```python
from build123d import *

# Parameters (mm, degrees)
F0_W     = 5.5
F0_H     = 3.5
F1_DEPTH = 4
F2_DEPTH = 8.5
F3_DEPTH = 1


with BuildPart() as f1:
    # F0 (on Front) → F1 (new body)
    with BuildSketch(Plane.XZ):
        Polygon((-5.5, 14.5), (-26.5, 14.5), (-26.5, -14.5), (26.5, -14.5), (26.5, 14.5), (5.5, 14.5), (5.5, 11), (23, 11), (23, -11), (-23, -11), (-23, 11), (-5.5, 11), align=None)
        with Locations((-2.75, 12.75)):
            Rectangle(F0_W, F0_H)
        with Locations((2.75, 12.75)):
            Rectangle(F0_W, F0_H)
        Polygon((0, 11), (-5.5, 11), (-5.5, 6), (5.5, 6), (5.5, 11), align=None)
    extrude(amount=F1_DEPTH)

    # F0 (on Front) → F2 (join)
    with BuildSketch(Plane.XZ):
        Polygon((-5.5, 6), (-5.5, 11), (-23, 11), (-23, -11), (23, -11), (23, 11), (5.5, 11), (5.5, 6), align=None)
    extrude(amount=F2_DEPTH)

    # F0 (on Front) → F3 (join)
    with BuildSketch(Plane.XZ):
        with Locations((-2.75, 12.75)):
            Rectangle(F0_W, F0_H)
        with Locations((2.75, 12.75)):
            Rectangle(F0_W, F0_H)
        Polygon((0, 11), (-5.5, 11), (-5.5, 6), (5.5, 6), (5.5, 11), align=None)
    extrude(amount=F3_DEPTH)


solid = f1.part
```
Can you work these out from the model? Positions are in its coordinate system, mm. A direction names the side the tool comes from. Round coordinates to 2 decimals unless told otherwise and drop trailing zeros. Loops run counter-clockwise (first coordinate to the right, second up) from the corner with the lowest first, then second, coordinate; pieces in that order, holes last.
Item 1: Suppose I cut it at C-C, the plane z = 9. Write out the boundary of the cut face in (x, y).
Item 2: Will these pins go through, and if not, where does the flat tip stop? pin 1 Ø1.3 at (x, y) = (-17.5, -6.5) entering from +Z; pin 2 Ø3.5 at (y, z) = (-6.5, 8) entering from -X; pin 3 Ø2 at (y, z) = (-6.5, 8.5) entering from +X.
Item 3: Which directions (+Z, -Z, +X, -X, +Y, -Y) give clear straight access to the entire face, cutting with the end or side of a thin tool? Please do faces 5 (the flat face through (0, -2, 14.5)), 6 (the flat face through (-14, -6, 11)), 7 (the flat face through (0, -6, 6)), 8 (the flat face through (23, -6, 0)), 9 (the flat face through (-23, -6, 0)).
Item 4: Suppose I cut it at A-A, the plane x = -16. Write out the boundary of the cut face in (y, z), then the cut area to 3 significant figures.
Item 5: If we mould it in two halves opening along X, with no side actions, what happens to faces 1 (the flat face through (5.5, -6, 9)), 2 (the flat face through (0, -6, -11)), 3 (the flat face through (-26.5, -2, 0)), 4 (the flat face through (-5.5, -6, 8))? For each: +X half, -X half, draft (parallel to the pull), parting line (faces both ways), or undercut.
Item 6: Please list where these lines run through material, in increasing order: L1, parallel to X at y = -6.5, z = 9.5; L2, parallel to Z at x = -19, y = -6.5; L3, parallel to Y at x = -15.5, z = 12.
Item 7: Suppose I cut it at B-B, the plane z = -6.25. Write out the boundary of the cut face in (x, y).
Reported:
1. outline: (-26.5, -4) - (-23, -4) - (-23, -8.5) - (-5.5, -8.5) - (-5.5, -4) - (5.5, -4) - (5.5, -8.5) - (23, -8.5) - (23, -4) - (26.5, -4) - (26.5, 0) - (-26.5, 0) - close
2. pin 1: stops at z = 11
2. pin 2: stops at x = -23
2. pin 3: stops at x = 23
3. face 5: +Z, +X, -X, +Y, -Y
3. face 6: +Z, +X, -X, -Y
3. face 7: +Z, -Y
3. face 8: +Z, -Z, +X, -Y
3. face 9: +Z, -Z, -X, -Y
4. outline: (-8.5, -11) - (-4, -11) - (-4, -14.5) - (0, -14.5) - (0, 14.5) - (-4, 14.5) - (-4, 11) - (-8.5, 11) - close
4. area: 215 mm2
5. face 1: undercut
5. face 2: draft
5. face 3: -X half
5. face 4: undercut
6. L1: x = -23 to -5.5, 5.5 to 23
6. L2: z = -11 to 11
6. L3: y = -4 to 0
7. outline: (-26.5, -4) - (-23, -4) - (-23, -8.5) - (23, -8.5) - (23, -4) - (26.5, -4) - (26.5, 0) - (-26.5, 0) - close
